The drawing under review shows one solid part. Ordinate dimensions are in mm from its lowest x, y, z. Round coordinates to 2 decimals unless told otherwise and drop trailing zeros. Order: outer loops, then holes, each group sorted by start corner. A loop starts at its lowest first (then second) coordinate and runs counter-clockwise, first axis right, second up. Notation, with made-up numbers: M 8.5,41.25 L 38.5,41.25 A28 ccw 38.5,59.25 Z; hole C -1,-36.75 d6. An arc over 180 degrees is marked long. Answer as a JSON object with one key per item and string values. Group by question number.
1) Consider section C-C, the plane z = 40. Write out the cut boundary in (x, y), then the cut area to 3 significant figures.
2) Insertion check: pin 1 Ø5.5 at (x, z) = (7, 73) entering from -Y. The pin has a flat end and moves straight along its axis. Give the tip position at first contact, or say it passes through.
3) Consider section D-D, the plane y = 4. Write out the cut boundary in (x, z), then the cut area to 3 significant figures.
4) To check wall thickness, follow line 1 (X direction, y = 7.5, z = 73); line 2 (Z direction, x = 7, y = 4.75); line 3 (Z direction, x = 8, y = 8.75). State the ranges of each line that lie inside material, in increasing order.
5) The part is to be moulded in two halves that separate along X. For the marked faces 1 and 2, say which applies: +X half, -X half, draft (parallel to the pull), parting line (faces both ways), or undercut.
6) Consider section A-A, the plane x = 20. Write out the cut boundary in (y, z).
7) Consider section B-B, the plane x = 7. Write out the cut boundary in (y, z), then the cut area to 3 significant figures.
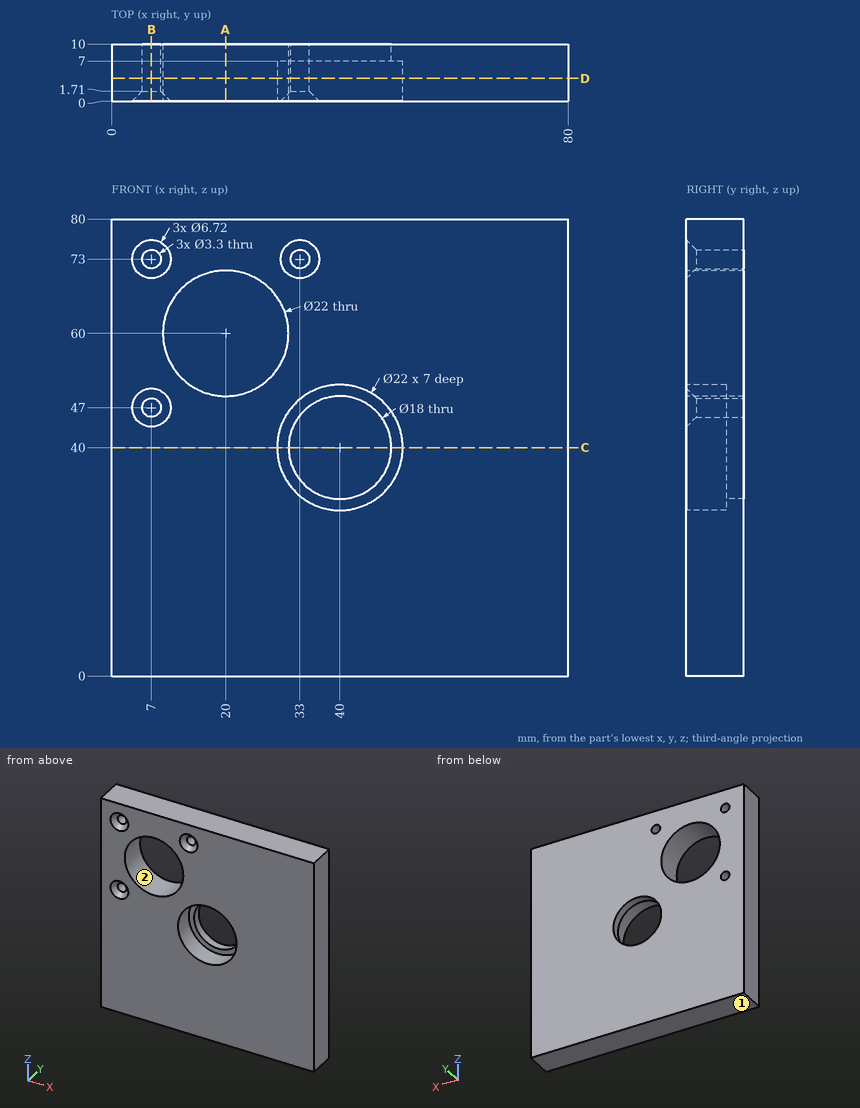
Results list:
{
 "1": {"outline": "M 0,0 L 29,0 L 29,7 L 31,7 L 31,10 L 0,10 Z; M 49,7 L 51,7 L 51,0 L 80,0 L 80,10 L 49,10 Z", "area": "592 mm^2"},
 "2": {"pin 1": "y = 0.61"},
 "3": {"outline": "M 0,0 L 80,0 L 80,80 L 0,80 Z; hole C 7,47 d3.3; hole C 7,73 d3.3; hole C 20,60 d22; hole C 40,40 d22; hole C 33,73 d3.3", "area": "5,610 mm^2"},
 "4": {"line 1": "0 to 5.35, 8.65 to 31.35, 34.65 to 80", "line 2": "0 to 45.35, 48.65 to 71.35, 74.65 to 80", "line 3": "0 to 45.69, 48.31 to 71.69, 74.31 to 80"},
 "5": {"face 1": "draft", "face 2": "undercut"},
 "6": {"outline": "M 0,0 L 10,0 L 10,49 L 0,49 Z; M 0,71 L 10,71 L 10,80 L 0,80 Z"},
 "7": {"outline": "M 0,0 L 10,0 L 10,45.35 L 1.71,45.35 L 0,43.64 Z; M 0,50.36 L 1.71,48.65 L 10,48.65 L 10,71.35 L 1.71,71.35 L 0,69.64 Z; M 0,76.36 L 1.71,74.65 L 10,74.65 L 10,80 L 0,80 Z", "area": "728 mm^2"}
}
